Geometry check sheet. Reference: the model listing, model coordinates, mm. Face numbers are marked on the shaded views. A direction names the side the tool comes from. Coordinates: 2 decimals unless noted, no trailing zeros. Write each loop counter-clockwise with the first axis right and the second up, starting at its lowest first coordinate (ties: lowest second). Pieces come first, ordered by that corner, then holes. Notation, with made-up numbers: (32.5, 15.5) - (41.5, 15.5) arc R21 ccw to (41.5, 41.5) - close; hole circle Ø1 at (78.5, 62.5). An arc over 180 degrees is marked (long way). Answer as a JSON object with one key per item and string values. Group by question number.
from build123d import *

# Parameters (mm, degrees)
F0_R          = 5
F1_DEPTH      = 10.2
F2_R          = 4.8
F3_DEPTH      = 3
F5_DEPTH      = 3
F5_DEPTH_BACK = 30
F6_R          = 2.5
F7_DEPTH      = 28


with BuildPart() as f1:
    # F0 (on Right) → F1 (new body)
    with BuildSketch(Plane.YZ):
        Circle(F0_R)
    extrude(amount=-F1_DEPTH)

    # F2 (on face) → F3 (join)
    with BuildSketch(Plane.YZ):
        Circle(F2_R)
    extrude(amount=F3_DEPTH)

    # F4 (on face) → F5 (join, two sides)
    with BuildSketch(Plane.YZ.offset(3)) as f5_sk:
        Polygon((-4.565071, -1.483282), (0, -4.8), (4.565071, -1.483282), (2.821369, 3.883282), (-2.821369, 3.883282), align=None)
    extrude(amount=F5_DEPTH)
    extrude(f5_sk.sketch, amount=-F5_DEPTH_BACK)

    # F6 (on face) → F7 (cut)
    with BuildSketch(Plane.YZ.offset(6)):
        Circle(F6_R)
    extrude(amount=-F7_DEPTH, mode=Mode.SUBTRACT)


solid = f1.part
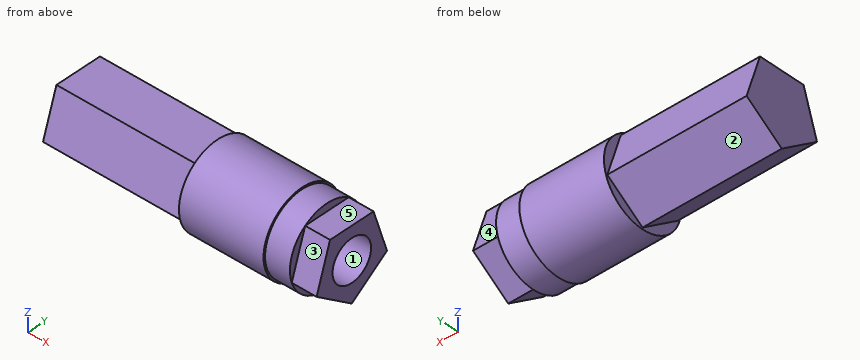
(1) Gauge pin test, flat ends, axial feed: pin 1 (2 mm diameter, centred on x = -9.5, y = 2, fed in from -Z); pin 2 (6 mm diameter, centred on x = -19.5, z = 3, fed in from +Y); pin 3 (3 mm diameter, centred on x = -14.5, z = 1.5, fed in from -Y). Record the tip position at first contact, or that the pin passes through.
(2) Material ranges on L1, parallel to Z at x = -2.5, y = 0; L2, parallel to X at y = 0, z = 0.25; L3, parallel to Y at x = -21.5, z = 2, recorded low to high. Write a range as [from, to].
(3) Section check D-D (x = -25). Record the cut outline in (y, z).
(4) Section check C-C (z = 0). Record the cut outline in (x, y).
(5) Section check A-A (x = -7.5). Record the cut outline in (y, z), and give its area (3 significant figures).
(6) Section check B-B (y = 0.5). Record the cut outline in (x, z).
(7) Set-up check for the marked faces 1, 2, 3, 4 and 5: record each of +Z, -Z, +X, -X, +Y, -Y from which the full face is reachable in a straight line by a thin tool's end or side.
Conclusion:
{
 "1": {"pin 1": "stops at z = -4.9", "pin 2": "stops at y = 4.08", "pin 3": "stops at y = -4.08"},
 "2": {"L1": "z = [-5, -2.5], [2.5, 5]", "L2": "x = [-27, -22]", "L3": "y = [-3.43, -1.5], [1.5, 3.43]"},
 "3": {"outline": "(-4.57, -1.48) - (0, -4.8) - (4.57, -1.48) - (2.82, 3.88) - (-2.82, 3.88) - close"},
 "4": {"outline": "(-27, -4.08) - (-10.2, -4.08) - (-10.2, -5) - (0, -5) - (0, -4.8) - (3, -4.8) - (3, -4.08) - (6, -4.08) - (6, -2.5) - (-22, -2.5) - (-22, 2.5) - (6, 2.5) - (6, 4.08) - (3, 4.08) - (3, 4.8) - (0, 4.8) - (0, 5) - (-10.2, 5) - (-10.2, 4.08) - (-27, 4.08) - close"},
 "5": {"outline": "circle Ø10 at (0, 0); hole circle Ø5 at (0, 0)", "area": "58.9 mm^2"},
 "6": {"outline": "(-27, -4.44) - (-10.2, -4.44) - (-10.2, -4.97) - (0, -4.97) - (0, -4.77) - (3, -4.77) - (3, -4.44) - (6, -4.44) - (6, -2.45) - (-22, -2.45) - (-22, 2.45) - (6, 2.45) - (6, 3.88) - (3, 3.88) - (3, 4.77) - (0, 4.77) - (0, 4.97) - (-10.2, 4.97) - (-10.2, 3.88) - (-27, 3.88) - close"},
 "7": {"face 1": "+X", "face 2": "-Z, -X, +Y", "face 3": "+Z, +X, -Y", "face 4": "+Z, +X, +Y", "face 5": "+Z, +X, +Y, -Y"}
}
